The figure shows three views and two pictorial views of one solid part (mm, origin at its lowest corner). Answer the questions. A direction names the side the tool comes from. Coordinates: 2 decimals unless noted, no trailing zeros. Write each loop counter-clockwise with the first axis right and the second up, starting at its lowest first coordinate (ties: lowest second). Pieces come first, ordered by that corner, then holes.
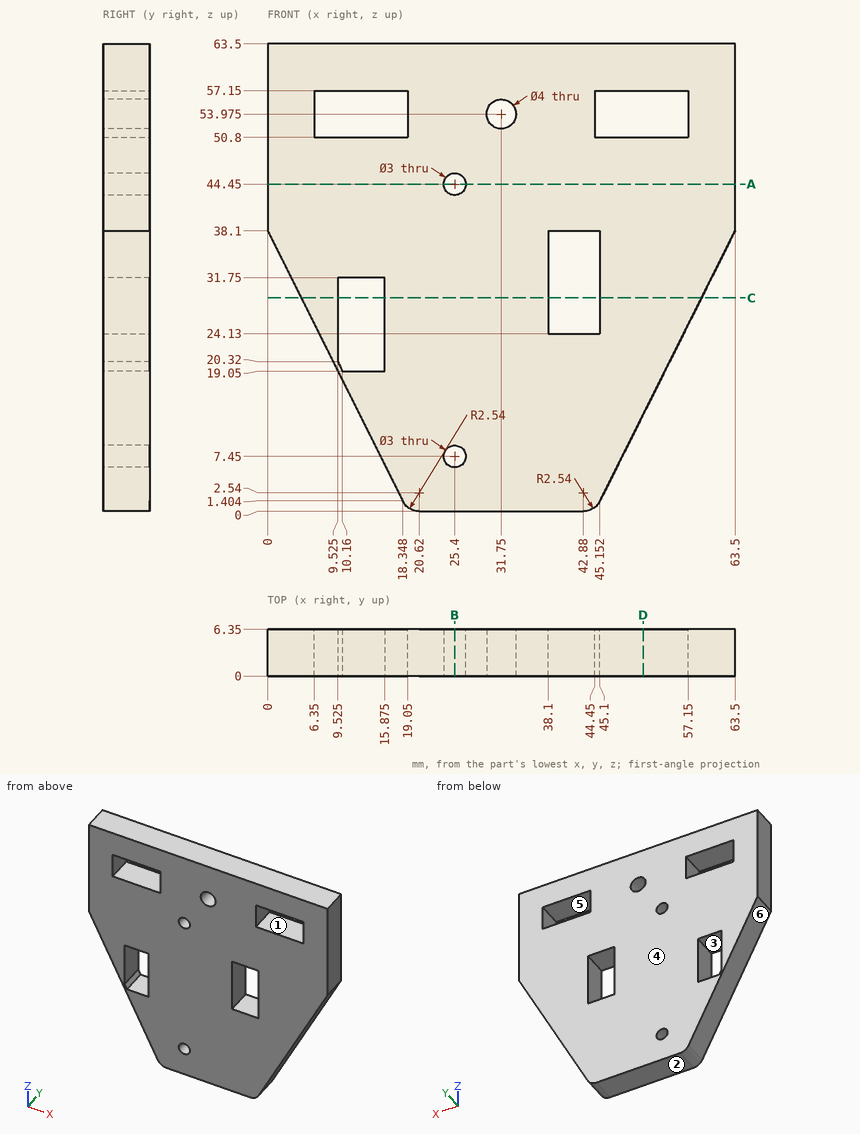
Q1. Find the intervals of material crossed by probe 1 along Z at (x, y) = (25.4, 1.75); probe 2 along Z at (x, y) = (31.75, 3.75) (3 decimals); probe 3 along Z at (x, y) = (26, 0.5) (1 decimal), in increasing order.
Answers below:
probe 1: z = 0 to 5.95, 8.95 to 42.95, 45.95 to 63.5
probe 2: z = 0 to 51.975, 55.975 to 63.5
probe 3: z = 0 to 6.1, 8.8 to 43.1, 45.8 to 63.5
Q2. Given pin 1 (2.5 mm diameter, centred on x = 25.4, z = 7.45, fed in from -Y); pin 2 (3 mm diameter, centred on y = 4, z = 25.5, fed in from +X); pin 3 (1.5 mm diameter, centred on y = 1.5, z = 12.5, fed in from -X) (1 decimal); pin 4 (5 mm diameter, centred on x = 7.5, z = 50, fed in from -Y), each flat-ended and moving along its own axis, determine where each tip first touches the part or whether it passes through.
Answers below:
pin 1: passes through
pin 2: stops at x = 57.95
pin 3: stops at x = 12.4
pin 4: stops at y = 0
Q3. The part is cut by section C-C, the plane z = 29. Write down the section's boundary in (x, y) (3 decimals).
Answers below:
outline: (4.55, 0) - (9.525, 0) - (9.525, 6.35) - (4.55, 6.35) - close; (15.875, 0) - (38.1, 0) - (38.1, 6.35) - (15.875, 6.35) - close; (45.1, 0) - (58.95, 0) - (58.95, 6.35) - (45.1, 6.35) - close
Q4. The part is cut by section A-A, the plane z = 44.45. Write down the section's boundary in (x, y).
Answers below:
outline: (0, 0) - (23.9, 0) - (23.9, 6.35) - (0, 6.35) - close; (26.9, 0) - (63.5, 0) - (63.5, 6.35) - (26.9, 6.35) - close
Q5. Determine the mould class of the marked faces 3, 4, 5 and 6 for opening direction X: released by +X, released by -X, zero draft, split by the parting line, or undercut.
Answers below:
face 3: undercut
face 4: zero draft
face 5: undercut
face 6: released by -X
Q6. Which of the six approach directions +Z, -Z, +X, -X, +Y, -Y give full straight-line access (tool end or side, diameter ignored) to the marked faces 1 and 2?
Answers below:
face 1: +Y, -Y
face 2: -Z, +X, -X, +Y, -Y
Q7. The part is cut by section D-D, the plane x = 51. Write down the section's boundary in (y, z), then the cut area to 3 significant figures.
Answers below:
outline: (0, 13.1) - (6.35, 13.1) - (6.35, 50.8) - (0, 50.8) - close; (0, 57.15) - (6.35, 57.15) - (6.35, 63.5) - (0, 63.5) - close
area: 280 mm2
Q8. The part is cut by section B-B, the plane x = 25.4. Write down the section's boundary in (y, z), then the cut area to 3 significant figures.
Answers below:
outline: (0, 0) - (6.35, 0) - (6.35, 5.95) - (0, 5.95) - close; (0, 8.95) - (6.35, 8.95) - (6.35, 42.95) - (0, 42.95) - close; (0, 45.95) - (6.35, 45.95) - (6.35, 63.5) - (0, 63.5) - close
area: 365 mm2
